Verification items for the finished model (mm, model axes). A direction names the side the tool comes from. Coordinates: 2 decimals unless noted, no trailing zeros. Order: outer loops, then holes, each group sorted by start corner. A loop starts at its lowest first (then second) coordinate and runs counter-clockwise, first axis right, second up. Notation, with made-up numbers: (40.25, 64.5) -> (84.25, 64.5) arc R27 cw to (84.25, 83.5) -> close; hole circle Ø6 at (73.5, 17.5). An arc over 180 degrees is marked (long way). Answer as CSV lines item,"result".
```python
from build123d import *

# Parameters (mm, degrees)
SKETCH_1_W      = 40
SKETCH_1_H      = 70
EXTRUDE_3_DEPTH = 50


with BuildPart() as part:
    # Эскиз1 → Бобышка-Вытянуть3 (new body)
    with BuildSketch(Plane.XY):
        with BuildLine():
            Line((-100, -215), (-200, -215))
            Line((-200, -215), (-200, -165))
            add(Edge.make_bspline(
                [(-200, 165), (-56.658015908, 0), (-200, -165)],
                knots=[0, 0, 0, 1, 1, 1], degree=2))
            Line((-200, 165), (-200, 215))
            Line((-200, 215), (0, 215))
            Line((0, 215), (200, 215))
            Line((200, 215), (200, 165))
            add(Edge.make_bspline(
                [(200, 165), (56.658015908, 0), (200, -165)],
                knots=[0, 0, 0, 1, 1, 1], degree=2))
            Line((200, -165), (200, -215))
            Line((200, -215), (100, -215))
            ThreePointArc((100, -215), (0, -115), (-100, -215))
        make_face()
        with Locations((0, 95)):
            Rectangle(SKETCH_1_W, SKETCH_1_H, mode=Mode.SUBTRACT)
    extrude(amount=EXTRUDE_3_DEPTH)


solid = part.part
```
Item 1: Section check B-B, the plane y = -178. Record the boundary of the cut face in (x, z).
Answer list:
outline,"(-200, 0) -> (-92.9, 0) -> (-92.9, 50) -> (-200, 50) -> close; (92.9, 0) -> (200, 0) -> (200, 50) -> (92.9, 50) -> close"
Item 2: Depth check by flat-ended pin: pin 1 Ø6 at (y, z) = (81, 36.5) entering from +X; pin 2 Ø20 at (x, z) = (5.5, 35) entering from -Y; pin 3 Ø25 at (y, z) = (95.5, 17) entering from +X (3 decimals). Enter the tip coordinate at first touch or a pass-through.
Answer list:
pin 1,"x = 146.9"
pin 2,"y = -116.21"
pin 3,"x = 159.035"
Item 3: Section check C-C, the plane x = -50. Record the boundary of the cut face in (y, z), plus the area to 3 significant figures.
Answer list:
outline,"(-128.4, 0) -> (215, 0) -> (215, 50) -> (-128.4, 50) -> close"
area,"17,200 mm2"
Item 4: Thickness scan on line 1 (Y direction, x = -4.5, z = 31); line 2 (Y direction, x = -159, z = 44); line 3 (X direction, y = -135, z = 26). Record the ranges inside material, lowest first.
Answer list:
line 1,"-115.1 to 60, 130 to 215"
line 2,"-215 to -107.94, 107.94 to 215"
line 3,"-176.31 to -60, 60 to 176.31"
Item 5: Tool access check on faces 1 (the flat face through (200, 190, 25)), 2 (the flat face through (-20, 95, 25)). Record the directions out of +Z, -Z, +X, -X, +Y, -Y that give a thin tool (end or side, any length) a straight path to the whole face; none if there is none.
Answer list:
face 1,"+Z, -Z, +X, +Y, -Y"
face 2,"+Z, -Z"
Item 6: Release check for a two-part mould opening along Y. For faces 3 (the flat face through (20, 95, 25)), 4 (the flat face through (-3, 215, 25)), 5 (the cylindrical face through (2.199, -115.024, 24.65)), 6 (the flat face through (3, 51, 50)) record: +Y half, -Y half, draft (parallel to the pull), parting line (faces both ways), or undercut.
Answer list:
face 3,"undercut"
face 4,"+Y half"
face 5,"-Y half"
face 6,"draft"
Item 7: Section check A-A, the plane x = 0. Record the boundary of the cut face in (y, z), plus the area to 3 significant figures.
Answer list:
outline,"(-115, 0) -> (60, 0) -> (60, 50) -> (-115, 50) -> close; (130, 0) -> (215, 0) -> (215, 50) -> (130, 50) -> close"
area,"13,000 mm2"
